from build123d import *

# Parameters (mm, degrees)
SKETCH1_R           = 1.75
BOSS_EXTRUDE1_DEPTH = 3
SKETCH2_R           = 1.5
BOSS_EXTRUDE2_DEPTH = 8
FILLET1_R           = 3.5
CUT_EXTRUDE1_DEPTH  = 4


with BuildPart() as part:
    # Sketch1 → Boss-Extrude1 (new body)
    with BuildSketch(Plane.XY):
        with BuildLine():
            Line((-20, 16), (-20, 14.466251376))
            ThreePointArc((-20, 14.466251376), (-19.517003263, 12.560814931), (-18.184655977, 11.115538278))
            ThreePointArc((-18.184655977, 11.115538278), (-14.41606767, 10.198360315), (-10.905843198, 11.848147392))
            ThreePointArc((-10.905843198, 11.848147392), (-9.615070973, 12.700850549), (-8.097274802, 13))
            Line((-8.097274802, 13), (12, 13))
            Line((12, 13), (12, -13))
            Line((12, -13), (-8.097274802, -13))
            ThreePointArc((-8.097274802, -13), (-9.615070973, -12.700850549), (-10.905843198, -11.848147392))
            ThreePointArc((-10.905843198, -11.848147392), (-14.41606767, -10.198360315), (-18.184655977, -11.115538278))
            ThreePointArc((-18.184655977, -11.115538278), (-19.517003263, -12.560814931), (-20, -14.466251376))
            Line((-20, -14.466251376), (-20, -16))
            ThreePointArc((-20, -16), (-18.535533906, -19.535533906), (-15, -21))
            Line((-15, -21), (12, -21))
            ThreePointArc((12, -21), (17.656854249, -18.656854249), (20, -13))
            Line((20, -13), (20, 13))
            ThreePointArc((20, 13), (17.656854249, 18.656854249), (12, 21))
            Line((12, 21), (-15, 21))
            ThreePointArc((-15, 21), (-18.535533906, 19.535533906), (-20, 16))
        make_face()
        with Locations((15, 15.5)):
            Circle(SKETCH1_R, mode=Mode.SUBTRACT)
        with Locations((15, -15.5)):
            Circle(SKETCH1_R, mode=Mode.SUBTRACT)
        with Locations((-16, -15.5)):
            Circle(SKETCH1_R, mode=Mode.SUBTRACT)
        with Locations((-16, 15.5)):
            Circle(SKETCH1_R, mode=Mode.SUBTRACT)
    extrude(amount=BOSS_EXTRUDE1_DEPTH)

    # Sketch2 → Boss-Extrude2 (add)
    with BuildSketch(Plane(origin=(20, 0, 0), x_dir=(0, 0, -1), z_dir=(1, 0, 0))):
        Polygon((-10.5, 3), (-7.5, 6), (-3, 6), (-3, -6), (-7.5, -6), (-10.5, -3), align=None)
        with Locations(Location((-6, 0, 0), (0, 0, 90))):
            Circle(SKETCH2_R, mode=Mode.SUBTRACT)
    extrude(amount=-BOSS_EXTRUDE2_DEPTH)

    # Fillet1
    fillet1_edges = [part.edges().sort_by_distance(p)[0] for p in [
        (16, 6, 3),
        (16, -6, 3),
        (12, -13, 1.5),
        (12, 13, 1.5),
    ]]
    fillet(fillet1_edges, radius=FILLET1_R - 0.0001)  # a hair under: the kernel refuses the full size

    # Sketch3 → Cut-Extrude1 (cut)
    with BuildSketch(Plane.ZY.offset(-12)):
        Polygon((6, 3.175426481), (3.25, 1.58771324), (3.25, -1.58771324), (6, -3.175426481), (8.75, -1.58771324), (8.75, 1.58771324), align=None)
    extrude(amount=-CUT_EXTRUDE1_DEPTH, mode=Mode.SUBTRACT)


solid = part.part
Geometry check sheet. Reference: the model listing, model coordinates, mm. A direction names the side the tool comes from. Round coordinates to 2 decimals unless told otherwise and drop trailing zeros. Write each loop counter-clockwise with the first axis right and the second up, starting at its lowest first coordinate (ties: lowest second). Pieces come first, ordered by that corner, then holes.
Item 1: Access from +Z, -Z, +X, -X, +Y, -Y to the whole of each face (thin tool, end or side, straight path). Record for faces 4 (the face through (-14.471, 10.193, 1.479)), 5 (the face through (13.972, 2.37, 7.394)), 6 (the face through (-19.504, -12.536, 1.479)).
Determined:
face 4: +Z, -Z
face 5: -X
face 6: +Z, -Z, -X
Item 2: Go/stop test with flat-tipped pins: pin 1 Ø3 at (x, y) = (-16, -15.5) entering from -Z; pin 2 Ø0.5 at (x, z) = (17, 7) entering from +Y; pin 3 Ø6 at (x, y) = (4, -16) entering from +Z; pin 4 Ø0.5 at (x, z) = (15.5, 7) entering from -Y. Record where each tip stops, or that it passes through.
Determined:
pin 1: passes through
pin 2: stops at y = 6
pin 3: stops at z = 3
pin 4: stops at y = -6
Item 3: Section check C-C (x = 15.5). Record the boundary of the cut face in (y, z).
Determined:
outline: (-20.19, 0) - (-17.18, 0) - (-17.18, 3) - (-20.19, 3) - close; (-13.82, 0) - (13.82, 0) - (13.82, 3) - (9.5, 3) arc R3.5 cw to (6, 6.5) - (6, 7.5) - (3, 10.5) - (-3, 10.5) - (-6, 7.5) - (-6, 6.5) arc R3.5 cw to (-9.5, 3) - (-13.82, 3) - close; (17.18, 0) - (20.19, 0) - (20.19, 3) - (17.18, 3) - close; hole (-3.18, 6) - (-1.59, 3.25) - (1.59, 3.25) - (3.18, 6) - (1.59, 8.75) - (-1.59, 8.75) - close
Item 4: Section check A-A (x = 8). Record the boundary of the cut face in (y, z).
Determined:
outline: (-21, 0) - (-13, 0) - (-13, 3) - (-21, 3) - close; (13, 0) - (21, 0) - (21, 3) - (13, 3) - close
Item 5: Section check B-B (y = -12.5). Record the boundary of the cut face in (x, z), plus the area to 3 significant figures.
Determined:
outline: (-19.48, 0) - (-10.03, 0) - (-10.03, 3) - (-19.48, 3) - close; (10.3, 0) - (20, 0) - (20, 3) - (10.3, 3) - close
area: 57.4 mm2
Item 6: Mould release check, pull along Z, two halves, no side actions. Record for faces 1 (the face through (0, -16, 3)), 2 (the face through (12, 0, 3)), 3 (the face through (14, 0, 8.75)): +Z half, -Z half, draft (parallel to the pull), parting line (faces both ways), or undercut.
Determined:
face 1: +Z half
face 2: draft
face 3: undercut
Item 7: Section check D-D (z = 2.25). Record the boundary of the cut face in (x, y), plus the area to 3 significant figures.
Determined:
outline: (-20, -16) arc R5 ccw to (-15, -21) - (12, -21) arc R8 ccw to (20, -13) - (20, 13) arc R8 ccw to (12, 21) - (-15, 21) arc R5 ccw to (-20, 16) - (-20, 14.47) arc R4 ccw to (-18.18, 11.12) arc R5.83 ccw to (-10.91, 11.85) arc R4 cw to (-8.1, 13) - (8.5, 13) arc R3.5 cw to (12, 9.5) - (12, -9.5) arc R3.5 cw to (8.5, -13) - (-8.1, -13) arc R4 cw to (-10.91, -11.85) arc R5.83 ccw to (-18.18, -11.12) arc R4 ccw to (-20, -14.47) - close; hole circle Ø3.5 at (-16, -15.5); hole circle Ø3.5 at (-16, 15.5); hole circle Ø3.5 at (15, -15.5); hole circle Ø3.5 at (15, 15.5)
area: 817 mm2
Item 8: Material ranges on line 1 along Y through (x, z) = (-16, 1); line 2 along Z through (x, y) = (18.95, 0); line 3 along X through (y, z) = (-4, 8), recorded low to high.
Determined:
line 1: y = -20.9 to -17.25, -13.75 to -10.26, 10.26 to 13.75, 17.25 to 20.9
line 2: z = 0 to 4.5, 7.5 to 10.5
line 3: x = 12 to 20
